Geometry check sheet. Reference: the model listing, model coordinates, mm. Face numbers are marked on the shaded views. Coordinates: 2 decimals unless noted, no trailing zeros. Write each loop counter-clockwise with the first axis right and the second up, starting at its lowest first coordinate (ties: lowest second). Pieces come first, ordered by that corner, then holes.
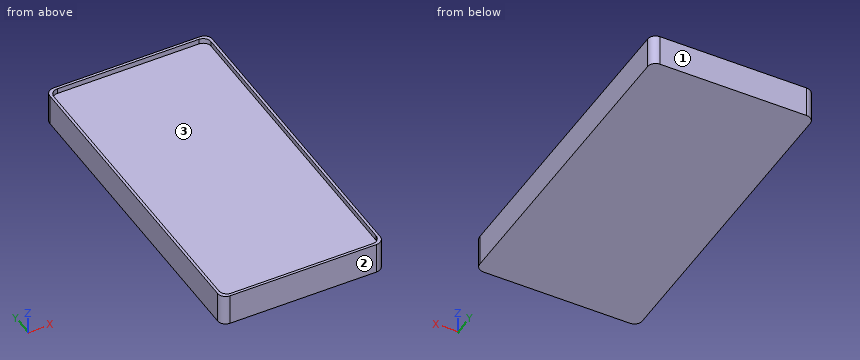
from build123d import *

# Parameters (mm, degrees)
SKETCH_1_W          = 615
SKETCH_1_H          = 1225
EXTRUDE_1_DEPTH     = 119
SKETCH_3_W          = 595
SKETCH_3_H          = 1205
CUT_EXTRUDE_1_DEPTH = 20
FILLET_3_R          = 30


with BuildPart() as part:
    # 스케치1 → 보스-돌출1 (new body)
    with BuildSketch(Plane.XY):
        with Locations((-307.5, 612.5)):
            Rectangle(SKETCH_1_W, SKETCH_1_H)
    extrude(amount=EXTRUDE_1_DEPTH)

    # 스케치3 → 컷-돌출1 (cut)
    with BuildSketch(Plane.XY.offset(119)):
        with Locations((-307.5, 612.5)):
            Rectangle(SKETCH_3_W, SKETCH_3_H)
    extrude(amount=-CUT_EXTRUDE_1_DEPTH, mode=Mode.SUBTRACT)

    # 필렛3
    fillet_3_edges = [part.edges().sort_by_distance(p)[0] for p in [
        (-10, 1215, 109),
        (-10, 10, 109),
        (-605, 10, 109),
        (-605, 1215, 109),
        (0, 0, 59.5),
        (-615, 0, 59.5),
        (-615, 1225, 59.5),
        (0, 1225, 59.5),
    ]]
    fillet(fillet_3_edges, radius=FILLET_3_R)


solid = part.part
1. Sectioned sample at B-B, the plane x = -469.5. Record the boundary of the cut face in (y, z), and give its area (3 significant figures).
Computed values:
outline: (0, 0) - (1225, 0) - (1225, 119) - (1215, 119) - (1215, 99) - (10, 99) - (10, 119) - (0, 119) - close
area: 122,000 mm2
2. Sectioned sample at A-A, the plane y = 912. Record the boundary of the cut face in (x, z).
Computed values:
outline: (-615, 0) - (0, 0) - (0, 119) - (-10, 119) - (-10, 99) - (-605, 99) - (-605, 119) - (-615, 119) - close
3. Draft check along Y on the marked faces 1, 2 and 3. Enter one of: released by +Y, released by -Y, zero draft, split by the parting line, or undercut.
Computed values:
face 1: released by +Y
face 2: released by -Y
face 3: undercut
4. Thickness scan on line 1 along X through (y, z) = (223, 106); line 2 along Z through (x, y) = (-253, 489.5); line 3 along Y through (x, z) = (-29.5, 17). Record the ranges inside material, lowest first.
Computed values:
line 1: x = -615 to -605, -10 to 0
line 2: z = 0 to 99
line 3: y = 0 to 1225
